Could you check a few things on this model? Use its own coordinates, in mm. Face numbers are marked on the shaded views. A direction names the side the tool comes from. Give positions to 0.01 mm unless a question says otherwise; leave off trailing zeros. Write each loop counter-clockwise with the first axis right and the second up, starting at its lowest first coordinate (ties: lowest second). Pieces come first, ordered by that corner, then holes. Notation, with made-up numbers: M 75,64.5 L 102,64.5 A32 cw 102,102.5 Z; hole C 60.25,-36 d4. An arc over 180 degrees is marked long. Use one line per item in the form item = value.
from build123d import *

# Parameters (mm, degrees)
SKETCH1_R           = 3.175
SKETCH1_R_2         = 3.96875
SKETCH1_R_3         = 2
BOSS_EXTRUDE1_DEPTH = 10.16


with BuildPart() as part:
    # Sketch1 → Boss-Extrude1 (new body)
    with BuildSketch(Plane(origin=(0, 0, 0), x_dir=(1, 0, 0), z_dir=(0, 1, 0))):
        with BuildLine():
            Line((54.2925, 31.75), (-12.3825, 31.75))
            Line((-12.3825, 31.75), (-12.3825, 13.97))
            Line((-12.3825, 13.97), (-6.35, 0))
            ThreePointArc((-6.35, 0), (0, -6.35), (6.35, 0))
            Line((6.35, 0), (35.56, 0))
            ThreePointArc((35.56, 0), (41.91, -6.35), (48.26, 0))
            Line((48.26, 0), (54.2925, 13.97))
            Line((54.2925, 13.97), (54.2925, 31.75))
        make_face()
        with Locations(Location((0, 0, 0), (0, 0, 270))):
            Circle(SKETCH1_R, mode=Mode.SUBTRACT)
        with Locations(Location((41.91, 0, 0), (0, 0, 270))):
            Circle(SKETCH1_R, mode=Mode.SUBTRACT)
        with Locations(Location((46.355, 22.86, 0), (0, 0, 270))):
            Circle(SKETCH1_R_2, mode=Mode.SUBTRACT)
        with Locations(Location((-4.445, 22.86, 0), (0, 0, 270))):
            Circle(SKETCH1_R_2, mode=Mode.SUBTRACT)
        with Locations(Location((11.43, 8.89, 0), (0, 0, 270))):
            Circle(SKETCH1_R_3, mode=Mode.SUBTRACT)
    extrude(amount=-BOSS_EXTRUDE1_DEPTH)


solid = part.part
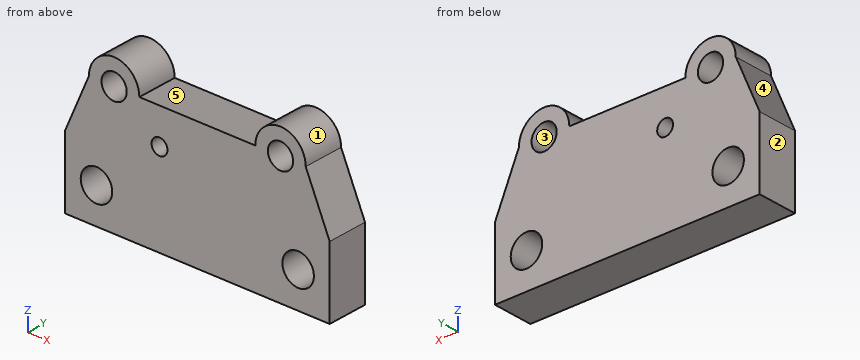
1) I want a section at A-A, the plane x = 11.43. Please give me the cut outline in (y, z), plus the area to 3 significant figures.
Checked values:
outline = M -10.16,-31.75 L 0,-31.75 L 0,-10.89 L -10.16,-10.89 Z; M -10.16,-6.89 L 0,-6.89 L 0,0 L -10.16,0 Z
area = 282 mm2
2) For the marked faces 4 and 5, which set-ups out of +Z, -Z, +X, -X, +Y, -Y let a thin tool reach every point of the face, with its end or its side?
Checked values:
face_4 = +Z, -X, +Y, -Y
face_5 = +Z, +Y, -Y
3) I want a section at C-C, the plane z = -8. Please give me the cut outline in (x, y).
Checked values:
outline = M -9.8,-10.16 L 9.64,-10.16 L 9.64,0 L -9.8,0 Z; M 13.22,-10.16 L 51.71,-10.16 L 51.71,0 L 13.22,0 Z
4) Thinking about a two-plate mould opening in Z: for the marked faces 1, 2 and 3, which applies, released by +Z, released by -Z, zero draft, split by the parting line, or undercut?
Checked values:
face_1 = released by +Z
face_2 = zero draft
face_3 = undercut
5) For pin 1 Ø6 at (y, z) = (-2, -8.5) entering from -X; pin 2 Ø1 at (y, z) = (-7, -7) entering from -X, each with a flat end and sliding along its axis, tell me the tip position at first contact or that it passes through.
Checked values:
pin_1 = -11.32
pin_2 = -9.59
6) I want a section at D-D, the plane y = -6.25. Count the separate pieces of the cut face and the enclosed holes in it, plus the area to 3 significant figures.
Checked values:
separate_pieces = 1
enclosed_holes = 5
area = 1,980 mm2
7) I want a section at B-B, the plane z = -22.86. Please give me the cut outline in (x, y), plus the area to 3 significant figures.
Checked values:
outline = M -12.38,-10.16 L -8.41,-10.16 L -8.41,0 L -12.38,0 Z; M -0.48,-10.16 L 42.39,-10.16 L 42.39,0 L -0.48,0 Z; M 50.32,-10.16 L 54.29,-10.16 L 54.29,0 L 50.32,0 Z
area = 516 mm2
8) If I drill on L1, parallel to X at y = -3.5, z = -22.86; L2, parallel to X at y = -7.75, z = -20.5; L3, parallel to Z at x = 16.5, y = -7.75, over which ranges is the centre line in solid material (lowest first)?
Checked values:
L1 = -12.38 to -8.41, -0.48 to 42.39, 50.32 to 54.29
L2 = -12.38 to -7.64, -1.25 to 43.16, 49.55 to 54.29
L3 = -31.75 to 0
